Source: CAD feature listing. Evaluate the final solid. Frame: model axes, mm. A direction names the side the tool comes from. Give positions to 0.01 mm unless a question says otherwise; leave off trailing zeros. Order: outer loops, then holes, each group sorted by start corner. A loop starts at its lowest first (then second) coordinate and runs counter-clockwise, first axis right, second up.
from build123d import *

# Parameters (mm, degrees)
SKETCH1_R           = 27
BOSS_EXTRUDE1_DEPTH = 60
SKETCH2_R           = 25.527
SKETCH2_R_2         = 22.0345
CUT_EXTRUDE1_DEPTH  = 1.9558
SKETCH3_R           = 2
CUT_EXTRUDE2_DEPTH  = 8
SKETCH8_R           = 3.4925
BOSS_EXTRUDE2_DEPTH = 63.5


with BuildPart() as part:
    # Sketch1 → Boss-Extrude1 (new body)
    with BuildSketch(Plane(origin=(0, 0, 0), x_dir=(1, 0, 0), z_dir=(0, 1, 0))):
        with Locations(Location((0, 0, 0), (0, 0, 270))):
            Circle(SKETCH1_R)
    extrude(amount=BOSS_EXTRUDE1_DEPTH)

    # Sketch2 → Cut-Extrude1 (cut)
    with BuildSketch(Plane.XZ):
        with Locations(Location((0, 0, 0), (0, 0, 270))):
            Circle(SKETCH2_R)
        with Locations(Location((0, 0, 0), (0, 0, 270))):
            Circle(SKETCH2_R_2, mode=Mode.SUBTRACT)
    extrude(amount=-CUT_EXTRUDE1_DEPTH, mode=Mode.SUBTRACT)

    # Sketch3 → Cut-Extrude2 (cut)
    with BuildSketch(Plane.XZ):
        with Locations(Location((0, 17, 0), (0, 0, 270))):
            Circle(SKETCH3_R)
        with Locations(Location((14.722431864, 8.5, 0), (0, 0, 270))):
            Circle(SKETCH3_R)
        with Locations(Location((14.722431864, -8.5, 0), (0, 0, 270))):
            Circle(SKETCH3_R)
        with Locations(Location((0, -17, 0), (0, 0, 270))):
            Circle(SKETCH3_R)
        with Locations(Location((-14.722431864, -8.5, 0), (0, 0, 270))):
            Circle(SKETCH3_R)
        with Locations(Location((-14.722431864, 8.5, 0), (0, 0, 270))):
            Circle(SKETCH3_R)
    extrude(amount=-CUT_EXTRUDE2_DEPTH, mode=Mode.SUBTRACT)

    # Loft1: read off the stored shape, not the designer's step
    # Loft1: loft between two sections, ruled curve by curve
    loft1_from = [
        Edge.make_bspline([(-3.433483362, -24.13, 0.639334225), (-2.154814912, -24.13, 7.50630095), (4.712151812, -24.13, 6.227632499), (3.433483362, -24.13, -0.639334225), (2.154814912, -24.13, -7.50630095), (-4.712151812, -24.13, -6.227632499), (-3.433483362, -24.13, 0.639334225)], [0, 0, 0, 0, 0.5, 0.5, 0.5, 1, 1, 1, 1], 3, [1, 0.333333333, 0.333333333, 1, 0.333333333, 0.333333333, 1]),
    ]
    loft1_to = [
        Edge.make_bspline([(0, 0, -7.62), (-15.24, 0, -7.62), (-15.24, 0, 7.62), (0, 0, 7.62), (15.24, 0, 7.62), (15.24, 0, -7.62), (0, 0, -7.62)], [0, 0, 0, 0, 0.5, 0.5, 0.5, 1, 1, 1, 1], 3, [1, 0.333333333, 0.333333333, 1, 0.333333333, 0.333333333, 1]),
    ]
    loft1 = Solid(Shell([*[Face.make_surface_from_curves(loft1_from[k], loft1_to[k]) for k in range(1)], Face(Wire(loft1_from)), Face(Wire(loft1_to))]))
    add(loft1)

    # Sketch8 → Boss-Extrude2 (add)
    with BuildSketch(Plane.XZ.offset(24.13)):
        with Locations(Location((0, 0, 0), (0, 0, 169.452))):
            Circle(SKETCH8_R)
    extrude(amount=BOSS_EXTRUDE2_DEPTH)


solid = part.part
(1) Section C-C, the plane z = -24. Return loops of the section in (x, y), plus the area to 3 significant figures.
(2) Section A-A, the plane z = 17. Return loops of the section in (x, y).
(3) Section B-B, the plane y = 25. Return loops of the section in (x, z).
(4) Section D-D, the plane y = -36. Return loops of the section in (x, z) (1 decimal), plus the area to 3 significant figures.
(5) Access query for faces 1 (the flat face through (0, 60, 0)), 2 (the cylindrical face through (12.77, 3.94, 8.93)). Directions: +Z, -Z, +X, -X, +Y, -Y. A direction counts if a zero-diameter tool reaches every point of the face in a straight line with its end or side. Return the directions, or none.
(6) Pin query (flat end, axial travel): pin 1 Ø3 at (x, z) = (14, -9) entering from -Y; pin 2 Ø10 at (y, z) = (2.5, 13) entering from -X; pin 3 Ø1.5 at (x, y) = (-20, 44.5) entering from -Z. Return the tip coordinate at first contact, or that it passes through.
(7) Line query: line 1 along X through (y, z) = (2, 8.5); line 2 along Y through (x, z) = (-21.5, -6); line 3 along Y through (x, z) = (1, 9). Output: solid intervals per line, ascending.
(8) Draft query along X for faces 3 (the flat face through (-10, 0, 24)), 4 (the cylindrical face through (-26.36, 29.58, -5.85)), 5 (the flat face through (-15, 8, -8)), 6 (the cylindrical face through (12.77, 3.94, -8.07)). Return one class per face: +X half, -X half, draft (parallel to the pull), parting line (faces both ways), or undercut.
Checks:
1. outline: (-12.37, 0) - (-8.7, 0) - (-8.7, 1.96) - (8.7, 1.96) - (8.7, 0) - (12.37, 0) - (12.37, 60) - (-12.37, 60) - close
1. area: 1,450 mm2
2. outline: (-20.98, 0) - (-19.04, 0) - (-19.04, 1.96) - (-14.02, 1.96) - (-14.02, 0) - (-2, 0) - (-2, 8) - (2, 8) - (2, 0) - (14.02, 0) - (14.02, 1.96) - (19.04, 1.96) - (19.04, 0) - (20.98, 0) - (20.98, 60) - (-20.98, 60) - close
3. outline: circle Ø54 at (0, 0)
4. outline: circle Ø7 at (0, 0)
4. area: 38.3 mm2
5. face 1: +Z, -Z, +X, -X, +Y
5. face 2: -Y
6. pin 1: stops at y = 0
6. pin 2: stops at x = -25.79
6. pin 3: stops at z = -18.93
7. line 1: x = -25.63 to -16.72, -12.72 to 12.72, 16.72 to 25.63
7. line 2: y = 1.96 to 60
7. line 3: y = 0 to 60
8. face 3: draft
8. face 4: parting line
8. face 5: undercut
8. face 6: undercut
